```python
from build123d import *

# Parameters (mm, degrees)
F1_DEPTH = 25.4


with BuildPart() as f1:
    # F0 (on Top) → F1 (new body)
    with BuildSketch(Plane.XY):
        with BuildLine():
            ThreePointArc((3.175, 27.119779), (1.590199, 27.258655), (0, 27.305))
            ThreePointArc((0, 27.305), (-1.590199, 27.258655), (-3.175, 27.119779))
            ThreePointArc((-3.175, 27.119779), (-5.326941, 26.780342), (-7.444973, 26.270428))
            ThreePointArc((-7.444973, 26.270428), (-10.449171, 25.226531), (-13.311608, 23.840389))
            ThreePointArc((-13.311608, 23.840389), (-15.169845, 22.703278), (-16.931515, 21.421643))
            ThreePointArc((-16.931515, 21.421643), (-19.307551, 19.307551), (-21.421643, 16.931515))
            ThreePointArc((-21.421643, 16.931515), (-22.703278, 15.169845), (-23.840389, 13.311608))
            ThreePointArc((-23.840389, 13.311608), (-25.226531, 10.449171), (-26.270428, 7.444973))
            ThreePointArc((-26.270428, 7.444973), (-26.780342, 5.326941), (-27.119779, 3.175))
            ThreePointArc((-27.119779, 3.175), (-27.305, 0), (-27.119779, -3.175))
            ThreePointArc((-27.119779, -3.175), (-26.780342, -5.326941), (-26.270428, -7.444973))
            ThreePointArc((-26.270428, -7.444973), (-25.226531, -10.449171), (-23.840389, -13.311608))
            ThreePointArc((-23.840389, -13.311608), (-22.703278, -15.169845), (-21.421643, -16.931515))
            ThreePointArc((-21.421643, -16.931515), (-19.307551, -19.307551), (-16.931515, -21.421643))
            ThreePointArc((-16.931515, -21.421643), (-15.169845, -22.703278), (-13.311608, -23.840389))
            ThreePointArc((-13.311608, -23.840389), (-10.449171, -25.226531), (-7.444973, -26.270428))
            ThreePointArc((-7.444973, -26.270428), (-5.326941, -26.780342), (-3.175, -27.119779))
            ThreePointArc((-3.175, -27.119779), (0, -27.305), (3.175, -27.119779))
            ThreePointArc((3.175, -27.119779), (5.326941, -26.780342), (7.444973, -26.270428))
            ThreePointArc((7.444973, -26.270428), (10.449171, -25.226531), (13.311608, -23.840389))
            ThreePointArc((13.311608, -23.840389), (15.169845, -22.703278), (16.931515, -21.421643))
            ThreePointArc((16.931515, -21.421643), (19.307551, -19.307551), (21.421643, -16.931515))
            ThreePointArc((21.421643, -16.931515), (22.703278, -15.169845), (23.840389, -13.311608))
            ThreePointArc((23.840389, -13.311608), (25.226531, -10.449171), (26.270428, -7.444973))
            ThreePointArc((26.270428, -7.444973), (26.780342, -5.326941), (27.119779, -3.175))
            ThreePointArc((27.119779, -3.175), (27.258655, -1.590199), (27.305, 0))
            ThreePointArc((27.305, 0), (27.258655, 1.590199), (27.119779, 3.175))
            ThreePointArc((27.119779, 3.175), (26.780342, 5.326941), (26.270428, 7.444973))
            ThreePointArc((26.270428, 7.444973), (25.226531, 10.449171), (23.840389, 13.311608))
            ThreePointArc((23.840389, 13.311608), (22.703278, 15.169845), (21.421643, 16.931515))
            ThreePointArc((21.421643, 16.931515), (19.307551, 19.307551), (16.931515, 21.421643))
            ThreePointArc((16.931515, 21.421643), (15.169845, 22.703278), (13.311608, 23.840389))
            ThreePointArc((13.311608, 23.840389), (10.449171, 25.226531), (7.444973, 26.270428))
            ThreePointArc((7.444973, 26.270428), (5.326941, 26.780342), (3.175, 27.119779))
        make_face()
        with BuildLine():
            ThreePointArc((7.9375, 0), (-5.61266, -5.61266), (0, 7.9375))
            ThreePointArc((0, 7.9375), (5.61266, 5.61266), (7.9375, 0))
        make_face(mode=Mode.SUBTRACT)
        with BuildLine():
            ThreePointArc((-13.311608, 23.840389), (-10.449171, 25.226531), (-7.444973, 26.270428))
            Line((-7.444973, 26.270428), (-8.780969, 29.49581))
            ThreePointArc((-8.780969, 29.49581), (-9.464382, 29.976089), (-10.298293, 29.927998))
            Line((-10.298293, 29.927998), (-13.849286, 28.457129))
            ThreePointArc((-13.849286, 28.457129), (-14.536605, 27.76981), (-14.536605, 26.797794))
            Line((-14.536605, 26.797794), (-13.311608, 23.840389))
        make_face()
        with BuildLine():
            ThreePointArc((-21.421643, 16.931515), (-19.307551, 19.307551), (-16.931515, 21.421643))
            Line((-16.931515, 21.421643), (-19.400115, 23.890243))
            ThreePointArc((-19.400115, 23.890243), (-20.215301, 24.072433), (-20.967332, 23.708879))
            Line((-20.967332, 23.708879), (-23.685143, 20.991067))
            ThreePointArc((-23.685143, 20.991067), (-24.057118, 20.093041), (-23.685143, 19.195015))
            Line((-23.685143, 19.195015), (-21.421643, 16.931515))
        make_face()
        with BuildLine():
            ThreePointArc((-26.270428, 7.444973), (-25.226531, 10.449171), (-23.840389, 13.311608))
            Line((-23.840389, 13.311608), (-27.06577, 14.647604))
            ThreePointArc((-27.06577, 14.647604), (-27.888625, 14.503968), (-28.444284, 13.880297))
            Line((-28.444284, 13.880297), (-29.915153, 10.329305))
            ThreePointArc((-29.915153, 10.329305), (-29.915153, 9.357289), (-29.227834, 8.66997))
            Line((-29.227834, 8.66997), (-26.270428, 7.444973))
        make_face()
        with BuildLine():
            ThreePointArc((-27.119779, -3.175), (-27.305, 0), (-27.119779, 3.175))
            Line((-27.119779, 3.175), (-30.610906, 3.175))
            ThreePointArc((-30.610906, 3.175), (-31.316158, 2.727404), (-31.590851, 1.938566))
            Line((-31.590851, 1.938566), (-31.590851, -1.905))
            ThreePointArc((-31.590851, -1.905), (-31.218877, -2.803026), (-30.320851, -3.175))
            Line((-30.320851, -3.175), (-27.119779, -3.175))
        make_face()
        with BuildLine():
            ThreePointArc((-23.840389, -13.311608), (-25.226531, -10.449171), (-26.270428, -7.444973))
            Line((-26.270428, -7.444973), (-29.49581, -8.780969))
            ThreePointArc((-29.49581, -8.780969), (-29.976089, -9.464382), (-29.927998, -10.298293))
            Line((-29.927998, -10.298293), (-28.457129, -13.849286))
            ThreePointArc((-28.457129, -13.849286), (-27.76981, -14.536605), (-26.797794, -14.536605))
            Line((-26.797794, -14.536605), (-23.840389, -13.311608))
        make_face()
        with BuildLine():
            ThreePointArc((-16.931515, -21.421643), (-19.307551, -19.307551), (-21.421643, -16.931515))
            Line((-21.421643, -16.931515), (-23.890243, -19.400115))
            ThreePointArc((-23.890243, -19.400115), (-24.072433, -20.215301), (-23.708879, -20.967332))
            Line((-23.708879, -20.967332), (-20.991067, -23.685143))
            ThreePointArc((-20.991067, -23.685143), (-20.093041, -24.057118), (-19.195015, -23.685143))
            Line((-19.195015, -23.685143), (-16.931515, -21.421643))
        make_face()
        with BuildLine():
            ThreePointArc((-7.444973, -26.270428), (-10.449171, -25.226531), (-13.311608, -23.840389))
            Line((-13.311608, -23.840389), (-14.647604, -27.06577))
            ThreePointArc((-14.647604, -27.06577), (-14.503968, -27.888625), (-13.880297, -28.444284))
            Line((-13.880297, -28.444284), (-10.329305, -29.915153))
            ThreePointArc((-10.329305, -29.915153), (-9.357289, -29.915153), (-8.66997, -29.227834))
            Line((-8.66997, -29.227834), (-7.444973, -26.270428))
        make_face()
        with BuildLine():
            ThreePointArc((3.175, -27.119779), (0, -27.305), (-3.175, -27.119779))
            Line((-3.175, -27.119779), (-3.175, -30.610906))
            ThreePointArc((-3.175, -30.610906), (-2.727404, -31.316158), (-1.938566, -31.590851))
            Line((-1.938566, -31.590851), (1.905, -31.590851))
            ThreePointArc((1.905, -31.590851), (2.803026, -31.218877), (3.175, -30.320851))
            Line((3.175, -30.320851), (3.175, -27.119779))
        make_face()
        with BuildLine():
            Line((14.536605, -26.797794), (13.311608, -23.840389))
            ThreePointArc((13.311608, -23.840389), (10.449171, -25.226531), (7.444973, -26.270428))
            Line((7.444973, -26.270428), (8.780969, -29.49581))
            ThreePointArc((8.780969, -29.49581), (9.464382, -29.976089), (10.298293, -29.927998))
            Line((10.298293, -29.927998), (13.849286, -28.457129))
            ThreePointArc((13.849286, -28.457129), (14.536605, -27.76981), (14.536605, -26.797794))
        make_face()
        with BuildLine():
            Line((23.685143, -19.195015), (21.421643, -16.931515))
            ThreePointArc((21.421643, -16.931515), (19.307551, -19.307551), (16.931515, -21.421643))
            Line((16.931515, -21.421643), (19.400115, -23.890243))
            ThreePointArc((19.400115, -23.890243), (20.215301, -24.072433), (20.967332, -23.708879))
            Line((20.967332, -23.708879), (23.685143, -20.991067))
            ThreePointArc((23.685143, -20.991067), (24.057118, -20.093041), (23.685143, -19.195015))
        make_face()
        with BuildLine():
            Line((29.227834, -8.66997), (26.270428, -7.444973))
            ThreePointArc((26.270428, -7.444973), (25.226531, -10.449171), (23.840389, -13.311608))
            Line((23.840389, -13.311608), (27.06577, -14.647604))
            ThreePointArc((27.06577, -14.647604), (27.888625, -14.503968), (28.444284, -13.880297))
            Line((28.444284, -13.880297), (29.915153, -10.329305))
            ThreePointArc((29.915153, -10.329305), (29.915153, -9.357289), (29.227834, -8.66997))
        make_face()
        with BuildLine():
            Line((30.320851, 3.175), (27.119779, 3.175))
            ThreePointArc((27.119779, 3.175), (27.258655, 1.590199), (27.305, 0))
            ThreePointArc((27.305, 0), (27.258655, -1.590199), (27.119779, -3.175))
            Line((27.119779, -3.175), (30.610906, -3.175))
            ThreePointArc((30.610906, -3.175), (31.316158, -2.727404), (31.590851, -1.938566))
            Line((31.590851, -1.938566), (31.590851, 1.905))
            ThreePointArc((31.590851, 1.905), (31.218877, 2.803026), (30.320851, 3.175))
        make_face()
        with BuildLine():
            Line((26.797794, 14.536605), (23.840389, 13.311608))
            ThreePointArc((23.840389, 13.311608), (25.226531, 10.449171), (26.270428, 7.444973))
            Line((26.270428, 7.444973), (29.49581, 8.780969))
            ThreePointArc((29.49581, 8.780969), (29.976089, 9.464382), (29.927998, 10.298293))
            Line((29.927998, 10.298293), (28.457129, 13.849286))
            ThreePointArc((28.457129, 13.849286), (27.76981, 14.536605), (26.797794, 14.536605))
        make_face()
        with BuildLine():
            Line((19.195015, 23.685143), (16.931515, 21.421643))
            ThreePointArc((16.931515, 21.421643), (19.307551, 19.307551), (21.421643, 16.931515))
            Line((21.421643, 16.931515), (23.890243, 19.400115))
            ThreePointArc((23.890243, 19.400115), (24.072433, 20.215301), (23.708879, 20.967332))
            Line((23.708879, 20.967332), (20.991067, 23.685143))
            ThreePointArc((20.991067, 23.685143), (20.093041, 24.057118), (19.195015, 23.685143))
        make_face()
        with BuildLine():
            Line((8.66997, 29.227834), (7.444973, 26.270428))
            ThreePointArc((7.444973, 26.270428), (10.449171, 25.226531), (13.311608, 23.840389))
            Line((13.311608, 23.840389), (14.647604, 27.06577))
            ThreePointArc((14.647604, 27.06577), (14.503968, 27.888625), (13.880297, 28.444284))
            Line((13.880297, 28.444284), (10.329305, 29.915153))
            ThreePointArc((10.329305, 29.915153), (9.357289, 29.915153), (8.66997, 29.227834))
        make_face()
        with BuildLine():
            Line((1.938566, 31.590851), (0, 31.590851))
            Line((0, 31.590851), (0, 27.305))
            ThreePointArc((0, 27.305), (1.590199, 27.258655), (3.175, 27.119779))
            Line((3.175, 27.119779), (3.175, 30.610906))
            ThreePointArc((3.175, 30.610906), (2.727404, 31.316158), (1.938566, 31.590851))
        make_face()
        with BuildLine():
            Line((0, 27.305), (0, 31.590851))
            Line((0, 31.590851), (-1.905, 31.590851))
            ThreePointArc((-1.905, 31.590851), (-2.803026, 31.218877), (-3.175, 30.320851))
            Line((-3.175, 30.320851), (-3.175, 27.119779))
            ThreePointArc((-3.175, 27.119779), (-1.590199, 27.258655), (0, 27.305))
        make_face()
    extrude(amount=F1_DEPTH)


solid = f1.part
```
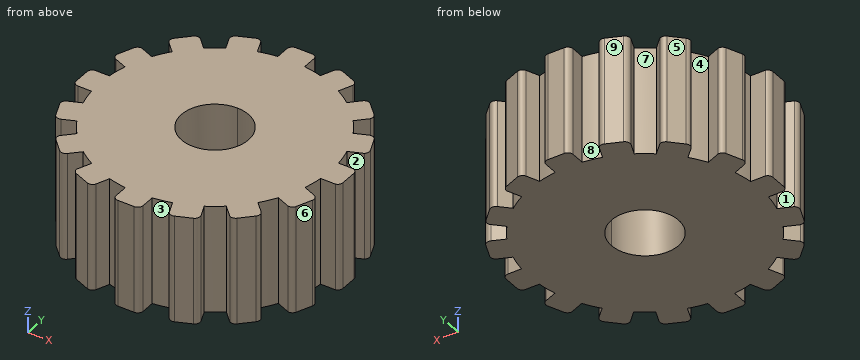
Read the model definition and answer for the solid it produces. Units are mm, in the model's axes. Face numbers are marked on the shaded views. A direction names the side the tool comes from. Coordinates: 2 decimals unless noted, no trailing zeros. Write each loop counter-clockwise with the first axis right and the second up, starting at its lowest first coordinate (ties: lowest second). Pieces come first, ordered by that corner, then holes. Notation, with made-up numbers: (83, 30) - (137, 30) arc R27 ccw to (137, 56) - close; hole circle Ø11 at (32.25, 86.5). An arc over 180 degrees is marked (long way). Answer as a JSON object with one key per item and string values. Group by question number.
1. The mould has two halves that part along X. Classify the marked faces 6, 7, 8 and 9: +X half, -X half, draft (parallel to the pull), parting line (faces both ways), or undercut.
2. A cutting plane is placed at B-B (y = -16). Determine the outline of the cut face in (x, z), plus the area to 3 significant figures.
3. A cutting plane is placed at A-A (x = 6.5). Determine the outline of the cut face in (y, z).
4. Consider L1, parallel to Y at x = 0, z = 9; L2, parallel to Y at x = 23.5, z = 13; L3, parallel to X at y = 22.5, z = 9.75. Determine where each line is inside the solid, lowest interval first. Write a range as [from, to].
5. Each of these flat-tipped pins is pushed along its axis until it touches: P1, Ø2, axis at y = 22.5, z = 9.5, coming from the -X side; P2, Ø1.6, axis at y = -28.5, z = 7.5, coming from the +X side; P3, Ø1.5, axis at x = -25, z = 6.5, coming from the +Y side; P4, Ø20.5, axis at x = 0, y = 0, coming from the +Z side. Where does it stop, or does it pass through?
6. Which of the six approach directions +Z, -Z, +X, -X, +Y, -Y give full straight-line access (tool end or side, diameter ignored) to the marked faces 1, 2, 3, 4 and 5?
Worked out:
{
 "1": {"face 6": "+X half", "face 7": "undercut", "face 8": "undercut", "face 9": "-X half"},
 "2": {"outline": "(-22.13, 0) - (22.13, 0) - (22.13, 25.4) - (-22.13, 25.4) - close", "area": "1,120 mm²"},
 "3": {"outline": "(-26.52, 0) - (-4.56, 0) - (-4.56, 25.4) - (-26.52, 25.4) - close; (4.56, 0) - (26.52, 0) - (26.52, 25.4) - (4.56, 25.4) - close"},
 "4": {"L1": "y = [-31.59, -7.94], [7.94, 31.59]", "L2": "y = [-21.18, -19.01], [-13.9, 13.9], [19.01, 21.18]", "L3": "x = [-22.18, -18.01], [-15.47, 15.47], [18.01, 22.18]"},
 "5": {"P1": "stops at x = -23.18", "P2": "stops at x = 14.56", "P3": "stops at y = 14.1", "P4": "stops at z = 25.4"},
 "6": {"face 1": "+Z, -Z, -X", "face 2": "+Z, -Z, +X", "face 3": "+Z, -Z, -Y", "face 4": "+Z, -Z", "face 5": "+Z, -Z, -X, +Y"}
}
